```python
from build123d import *

# Parameters (mm, degrees)
SKETCH_1_R      = 1.65
EXTRUDE_1_DEPTH = 5
SKETCH_2_W      = 44
SKETCH_2_H      = 20
SKETCH_2_R      = 1.6
EXTRUDE_2_DEPTH = 4
EXTRUDE_4_DEPTH = 3
EXTRUDE_5_DEPTH = 3
EXTRUDE_6_DEPTH = 3


with BuildPart() as part:
    # 草图1 → 凸台-拉伸1 (new body)
    with BuildSketch(Plane(origin=(0, 0, 0), x_dir=(1, 0, 0), z_dir=(0, 1, 0))):
        Polygon((-20, 20), (20, 20), (20, -20), (11, -20), (11, 16), (-11, 16), (-11, -20), (-20, -20), align=None)
        with Locations(Location((-13.5, -15.5, 0), (0, 0, 270))):
            Circle(SKETCH_1_R, mode=Mode.SUBTRACT)
        with Locations(Location((13.5, -15.5, 0), (0, 0, 90))):
            Circle(SKETCH_1_R, mode=Mode.SUBTRACT)
        with Locations(Location((13.5, 11.5, 0), (0, 0, 270))):
            Circle(SKETCH_1_R, mode=Mode.SUBTRACT)
        with Locations(Location((-13.5, 11.5, 0), (0, 0, 90))):
            Circle(SKETCH_1_R, mode=Mode.SUBTRACT)
    extrude(amount=EXTRUDE_1_DEPTH)

    # 草图2 → 凸台-拉伸2 (add)
    with BuildSketch(Plane(origin=(0, 0, -20), x_dir=(-1, 0, 0), z_dir=(0, 0, -1))):
        with Locations((0, 10)):
            Rectangle(SKETCH_2_W, SKETCH_2_H)
        with Locations((-15.5, 12)):
            Circle(SKETCH_2_R, mode=Mode.SUBTRACT)
        with Locations(Location((15.5, 12, 0), (0, 0, 180))):
            Circle(SKETCH_2_R, mode=Mode.SUBTRACT)
    extrude(amount=-EXTRUDE_2_DEPTH)

    # 草图4 → 凸台-拉伸4 (add)
    with BuildSketch(Plane.ZY.offset(20)):
        Polygon((-16, 0), (-6, 5), (-16, 5), align=None)
    extrude(amount=-EXTRUDE_4_DEPTH)

    # 草图5 → 凸台-拉伸5 (add)
    with BuildSketch(Plane(origin=(20, 0, 0), x_dir=(0, 0, -1), z_dir=(1, 0, 0))):
        Polygon((16, 10), (6, 5), (16, 5), align=None)
    extrude(amount=-EXTRUDE_5_DEPTH)

    # 草图6 → 凸台-拉伸6 (add)
    with BuildSketch(Plane.ZY.offset(20)):
        Polygon((-16, 10), (-16, 5), (-6, 5), align=None)
    extrude(amount=-EXTRUDE_6_DEPTH)


solid = part.part
```
The listing builds one solid part. Answer for the finished solid, in the listing's coordinates (mm). A direction names the side the tool comes from. Give positions to 0.01 mm unless a question says otherwise; leave off trailing zeros. Loops run counter-clockwise (first coordinate to the right, second up) from the corner with the lowest first, then second, coordinate; pieces in that order, holes last. Notation, with made-up numbers: M 13,-26 L 30,-26 A8 ccw 30,-18 Z; hole C 23,52 d11. An arc over 180 degrees is marked long. One line per item, written item: value.
Q1. A cutting plane is placed at C-C on y = 12. Determine the outline of the cut face in (x, z), then the cut area to 3 significant figures.
Working result:
outline: M -22,-20 L -17.1,-20 L -17.1,-16 L -22,-16 Z; M -13.9,-20 L 13.9,-20 L 13.9,-16 L -13.9,-16 Z; M 17.1,-20 L 22,-20 L 22,-16 L 17.1,-16 Z
area: 150 mm^2
Q2. Determine the mould class of faces 4 (the face through (-13.004, 2.465, 17.074)), 5 (the face through (-18.521, 7.465, -10.93)), 6 (the face through (-17, 6, -13)) for opening direction Z: +Z half, -Z half, draft (parallel to the pull), parting line (faces both ways), or undercut.
Working result:
face 4: undercut
face 5: +Z half
face 6: draft
Q3. A cutting plane is placed at A-A on z = -7. Determine the outline of the cut face in (x, y), then the cut area to 3 significant figures.
Working result:
outline: M -20,0 L -11,0 L -11,5 L -17,5 L -17,5.5 L -20,5.5 Z; M 11,0 L 20,0 L 20,5.5 L 17,5.5 L 17,5 L 11,5 Z
area: 93.0 mm^2
Q4. A cutting plane is placed at B-B on z = -11.5. Determine the outline of the cut face in (x, y), then the cut area to 3 significant figures.
Working result:
outline: M -20,0 L -15.15,0 L -15.15,5 L -17,5 L -17,7.75 L -20,7.75 Z; M -11.85,0 L -11,0 L -11,5 L -11.85,5 Z; M 11,0 L 11.85,0 L 11.85,5 L 11,5 Z; M 15.15,0 L 20,0 L 20,7.75 L 17,7.75 L 17,5 L 15.15,5 Z
area: 73.5 mm^2
Q5. A cutting plane is placed at D-D on y = 4.25. Determine the outline of the cut face in (x, z), then the cut area to 3 significant figures.
Working result:
outline: M -22,-20 L 22,-20 L 22,-16 L 20,-16 L 20,20 L 11,20 L 11,-16 L -11,-16 L -11,20 L -20,20 L -20,-16 L -22,-16 Z; hole C -13.5,-11.5 d3.3; hole C -13.5,15.5 d3.3; hole C 13.5,-11.5 d3.3; hole C 13.5,15.5 d3.3
area: 790 mm^2
Q6. Find the intervals of material crossed by line 1 (X direction, y = 3.7, z = -11.5); line 2 (Y direction, x = -15.5, z = -17.2); line 3 (Y direction, x = 12.5, z = 1), in increasing order. Write a range as from..to.
Working result:
line 1: x = -20..-15.15, -11.85..-11, 11..11.85, 15.15..20
line 2: y = 0..10.4, 13.6..20
line 3: y = 0..5
Q7. For faces 1 (the face through (20, 3, -2)), 2 (the face through (0, 10, -16)), 3 (the face through (11, 2, 2)), determine the directions among +Z, -Z, +X, -X, +Y, -Y from which every point of the face is accessible in a straight line to the end or side of a thin tool.
Working result:
face 1: +Z, +X, +Y, -Y
face 2: +Z, +Y
face 3: +Z, +Y, -Y
Q8. Flat-ended cylindrical pins translate along their axes: P1, Ø4, axis at y = 3, z = 2.5, coming from the -X side; P2, Ø1, axis at y = 2.5, z = -12, coming from the +X side; P3, Ø4.5, axis at x = 13.5, z = -11.5, coming from the +Y side; P4, Ø3.5, axis at x = 15.5, y = 12, coming from the -Z side. Find the tip coordinate at first contact, or state that the pin passes through.
Working result:
P1: stops at x = -20
P2: stops at x = 20
P3: stops at y = 5
P4: stops at z = -20
